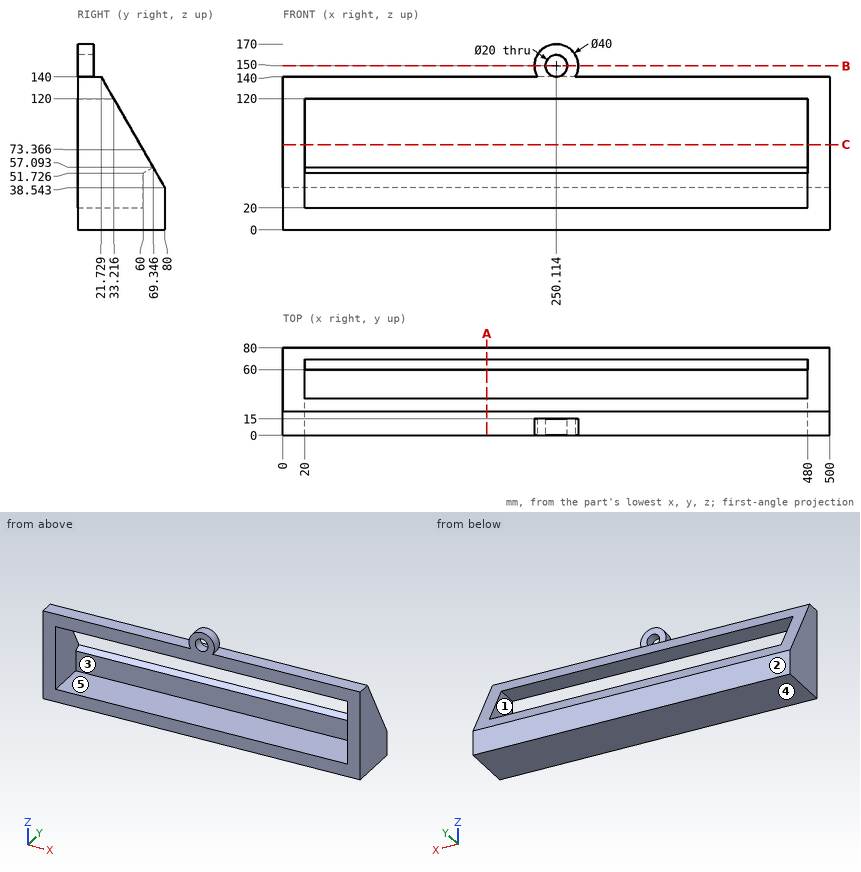
Check sheet for the drawn part. Datum: minimum x, y, z corner. Units: mm. A direction names the side the tool comes from. Give positions to 0.01 mm unless a question says otherwise; leave off trailing zeros. Order: outer loops, then holes, each group sorted by start corner. A loop starts at its lowest first (then second) coordinate and runs counter-clockwise, first axis right, second up. Notation, with made-up numbers: (29.5, 45.25) - (58.5, 45.25) arc R14 ccw to (58.5, 68.25) - close; hole circle Ø11 at (40, 40.25). An arc over 180 degrees is marked (long way). Answer as a JSON object with one key per item and string values.
(1) Tool access check on the marked faces 1 and 2. Record the directions out of +Z, -Z, +X, -X, +Y, -Y that give a thin tool (end or side, any length) a straight path to the whole face; none if there is none.
Report:
{"face 1": "-Y", "face 2": "+Z, -Z, +X, -X, +Y"}
(2) Draft check along Z on the marked faces 3, 4 and 5. Enter one of: released by +Z, released by -Z, zero draft, split by the parting line, or undercut.
Report:
{"face 3": "zero draft", "face 4": "released by -Z", "face 5": "undercut"}
(3) Depth check by flat-ended pin: pin 1 Ø4 at (x, z) = (323.5, 36.5) entering from -Y; pin 2 Ø10 at (x, y) = (357, 70) entering from +Z; pin 3 Ø23 at (x, z) = (250.11, 150) entering from +Y; pin 4 Ø12 at (x, z) = (195, 148) entering from -Y. Enter the tip coordinate at first touch or a pass-through.
Report:
{"pin 1": "y = 60", "pin 2": "z = 57.09", "pin 3": "y = 22.59", "pin 4": "through"}
(4) Cross-section at A-A (x = 186.5). Record the cut outline in (y, z) (1 decimal).
Report:
{"outline": "(0, 0) - (80, 0) - (80, 38.5) - (69.3, 57.1) - (60, 51.7) - (60, 20) - (0, 20) - close; (0, 120) - (33.2, 120) - (21.7, 140) - (0, 140) - close"}
(5) Material ranges on line 1 (X direction, y = 58.5, z = 65.5); line 2 (Z direction, x = 345.5, y = 18.5); line 3 (X direction, y = 10, z = 150), recorded low to high.
Report:
{"line 1": "0 to 20, 480 to 500", "line 2": "0 to 20, 120 to 140", "line 3": "230.11 to 240.11, 260.11 to 270.11"}
(6) Cross-section at B-B (z = 150). Record the cut outline in (x, y), then the cut area to 3 significant figures.
Report:
{"outline": "(230.11, 0) - (240.11, 0) - (240.11, 15) - (230.11, 15) - close; (260.11, 0) - (270.11, 0) - (270.11, 15) - (260.11, 15) - close", "area": "300 mm^2"}
(7) Cross-section at C-C (z = 78). Record the cut outline in (x, y), then the cut area to 3 significant figures.
Report:
{"outline": "(0, 0) - (20, 0) - (20, 57.34) - (0, 57.34) - close; (480, 0) - (500, 0) - (500, 57.34) - (480, 57.34) - close", "area": "2,290 mm^2"}
